from build123d import *

# Parameters (mm, degrees)
SKETCH1_R            = 2.5
BOSS_EXTRUDE1_DEPTH  = 30
SKETCH2_R            = 0.825
CUT_EXTRUDE1_DEPTH   = 5
CUT_EXTRUDE2_DEPTH   = 31.207614934
FILLET1_R            = 0.5
FILLET1_OF_MIRROR1_R = 0.5


with BuildPart() as part:
    # Sketch1 → Boss-Extrude1 (new body)
    with BuildSketch(Plane(origin=(0, 0, 0), x_dir=(1, 0, 0), z_dir=(0, 1, 0))):
        with Locations(Location((0, 0, 0), (0, 0, 270))):
            Circle(SKETCH1_R)
    boss_extrude1 = extrude(amount=BOSS_EXTRUDE1_DEPTH)

    # Sketch2 → Cut-Extrude1 (cut)
    with BuildSketch(Plane(origin=(0, 30, 0), x_dir=(1, 0, 0), z_dir=(0, 1, 0))):
        with Locations(Location((0, 0, 0), (0, 0, 270))):
            Circle(SKETCH2_R)
    cut_extrude1 = extrude(amount=-CUT_EXTRUDE1_DEPTH, mode=Mode.SUBTRACT)

    # Sketch3 → Cut-Extrude2 (cut, through all)
    with BuildSketch(Plane(origin=(0, 30, 0), x_dir=(1, 0, 0), z_dir=(0, 1, 0))):
        with BuildLine():
            Line((2, 1.5), (2, -1.5))
            ThreePointArc((2, -1.5), (2.5, 0), (2, 1.5))
        make_face()
    cut_extrude2 = extrude(amount=-CUT_EXTRUDE2_DEPTH, mode=Mode.SUBTRACT)

    # Fillet1
    fillet1_edges = [part.edges().sort_by_distance(p)[0] for p in [
        (-2.5, 30, 0),
    ]]
    fillet(fillet1_edges, radius=FILLET1_R - 0.0001)  # a hair under: the kernel refuses the full size

    # Mirror1: Boss-Extrude1, Cut-Extrude1, Cut-Extrude2 across plane
    add(boss_extrude1.mirror(Plane.ZX))
    add(cut_extrude1.mirror(Plane.ZX), mode=Mode.SUBTRACT)
    add(cut_extrude2.mirror(Plane.ZX), mode=Mode.SUBTRACT)

    # Fillet1 of Mirror1
    fillet1_of_mirror1_edges = [part.edges().sort_by_distance(p)[0] for p in [
        (-2.5, -30, 0),
    ]]
    fillet(fillet1_of_mirror1_edges, radius=FILLET1_OF_MIRROR1_R - 0.0001)  # a hair under: the kernel refuses the full size


solid = part.part
CAD build for the part. Positions are in the model's coordinates, mm. A direction names the side the tool comes from. Round coordinates to 2 decimals unless told otherwise and drop trailing zeros. Loops run counter-clockwise (first coordinate to the right, second up) from the corner with the lowest first, then second, coordinate; pieces in that order, holes last.
(1) Drop flat-ended pins along their axis: pin 1 (2 mm diameter, centred on y = -23, z = -1.5, fed in from -X); pin 2 (1 mm diameter, centred on x = 0, z = 0, fed in from +Y). Give the stop position or say it passes through.
(2) Wall check: line 1 along X through (y, z) = (-26.8, 0) (3 decimals); line 2 along X through (y, z) = (-21, -0.2); line 3 along Y through (x, z) = (-0.5, 0.05). Give the ranges that are in metal, low to high.
(3) Two-plate mould, pull along X, no slides. Class faces 1 (the flat face through (-1, 30, 0)), 2 (the flat face through (2, 0, 0)), 3 (the flat face through (0, 25, 0)): +X half, -X half, draft (parallel to the pull), parting line (faces both ways), or undercut.
(4) Cut at B-B (y = 1.5). Give the cut face in (x, z).
(5) Which spindle directions (+Z, -Z, +X, -X, +Y, -Y) get a long thin tool onto all of the face, cutting with end or side? Do faces 4 (the flat face through (0, -25, 0)), 5 (the cylindrical face through (-0.502, 27.535, -0.655)), 6 (the cylindrical face through (-2.5, 0.4, -0.1)). Say none if no direction does.
(6) Cut at A-A (x = 0). Give the cut face in (y, z) (3 decimals).
Findings below:
1. pin 1: stops at x = -2.45
1. pin 2: stops at y = 25
2. line 1: x = -2.5 to -0.825, 0.825 to 2
2. line 2: x = -2.49 to 2
2. line 3: y = -25 to 25
3. face 1: draft
3. face 2: +X half
3. face 3: undercut
4. outline: (2, -1.5) - (2, 1.5) arc R2.5 ccw (long way) to start
5. face 4: -Y
5. face 5: +Y
5. face 6: +Y, -Y
6. outline: (-30, -2) arc R0.5 ccw to (-29.5, -2.5) - (29.5, -2.5) arc R0.5 ccw to (30, -2) - (30, -0.825) - (25, -0.825) - (25, 0.825) - (30, 0.825) - (30, 2) arc R0.5 ccw to (29.5, 2.5) - (-29.5, 2.5) arc R0.5 ccw to (-30, 2) - (-30, 0.825) - (-25, 0.825) - (-25, -0.825) - (-30, -0.825) - close
